Input: part model. Units: mm. Frame: model coordinates. Face numbers are marked on the shaded views. A direction names the side the tool comes from. Give positions to 0.01 mm unless a question says otherwise; leave off trailing zeros. Write each loop counter-clockwise with the first axis right and the second up, starting at its lowest first coordinate (ties: lowest second). Pieces come first, ordered by that corner, then holes. Notation, with made-up numbers: (-11.5, -4.75) -> (22.5, -4.75) arc R5 ccw to (22.5, 3.25) -> close; hole circle Ø1 at (57.25, 69.5). An arc over 180 degrees is marked (long way). Return JSON: item names as keys, results as strings. Group by question number.
Item 1: Section B-B, the plane x = 1.5. Return loops of the section in (y, z), then the cut area to 3 significant figures.
Item 2: Section D-D, the plane y = -15. Return loops of the section in (x, z), then the cut area to 3 significant figures.
Item 3: Pin query (flat end, axial travel): P1, Ø1.2, axis at y = -24, z = 3, coming from the +X side; P2, Ø0.8, axis at y = -27, z = 5.5, coming from the +X side; P3, Ø0.5, axis at x = 25, z = 5.5, coming from the -Y side; P4, Ø3, axis at x = 26, y = -1, coming from the -Z side. Return the tip coordinate at first contact, or that it passes through.
Item 4: Section C-C, the plane x = 24. Return loops of the section in (y, z), then the cut area to 3 significant figures.
Item 5: Set-up query: the marked faces 1 and 2. Return all of +Z, -Z, +X, -X, +Y, -Y with unobstructed straight access to the full face (end or side cutting, diameter ignored); none if empty.
Item 6: Section A-A, the plane z = 3.55. Return loops of the section in (x, y).
Item 7: Line query: line 1 (X direction, y = 0.5, z = 4.8); line 2 (Z direction, x = 10, y = -20); line 3 (Y direction, x = 28, z = 3.15). Output: solid intervals per line, ascending. Write a range as [from, to].
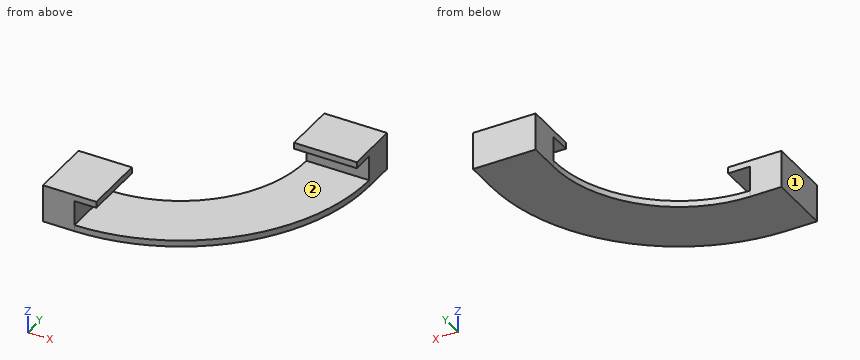
from build123d import *

# Parameters (mm, degrees)
F1_DEPTH = 1
F2_W     = 10
F2_H     = 5
F2_W_2   = 5
F2_H_2   = 10
F3_DEPTH = 5
F5_W     = 10
F5_H     = 1
F6_DEPTH = 3.5
F4_W     = 10
F4_H     = 1
F7_DEPTH = 3.5


with BuildPart() as f1:
    # F0 (on Top) → F1 (new body)
    with BuildSketch(Plane.XY):
        with BuildLine():
            Line((30, 0), (20, 0))
            ThreePointArc((20, 0), (14.1421356237, -14.1421356237), (0, -20))
            Line((0, -20), (0, -25))
            Line((0, -25), (0, -30))
            ThreePointArc((0, -30), (21.2132034356, -21.2132034356), (30, 0))
        make_face()
        with BuildLine():
            Line((20, 5), (20, 0))
            Line((20, 0), (30, 0))
            ThreePointArc((30, 0), (29.8949156836, 2.5087878084), (29.5803989155, 5))
            Line((29.5803989155, 5), (20, 5))
        make_face()
        with BuildLine():
            Line((0, -25), (0, -20))
            Line((0, -20), (-5, -20))
            Line((-5, -20), (-5, -29.5803989155))
            ThreePointArc((-5, -29.5803989155), (-2.5087878084, -29.8949156836), (0, -30))
            Line((0, -30), (0, -25))
        make_face()
        with BuildLine():
            ThreePointArc((29.5803989155, 5), (29.8949156836, 2.5087878084), (30, 0))
            Line((30, 0), (30, 5))
            Line((30, 5), (29.5803989155, 5))
        make_face()
        with BuildLine():
            Line((-5, -30), (0, -30))
            ThreePointArc((0, -30), (-2.5087878084, -29.8949156836), (-5, -29.5803989155))
            Line((-5, -29.5803989155), (-5, -30))
        make_face()
    extrude(amount=F1_DEPTH)

    # F2 (on face) → F3 (join)
    with BuildSketch(Plane.XY.offset(1)):
        with Locations((25, 2.5)):
            Rectangle(F2_W, F2_H)
        with Locations((-2.5, -25)):
            Rectangle(F2_W_2, F2_H_2)
    extrude(amount=F3_DEPTH)

    # F5 (on face) → F6 (join)
    with BuildSketch(Plane.YZ):
        with Locations((-25, 5.5)):
            Rectangle(F5_W, F5_H)
    extrude(amount=F6_DEPTH)

    # F4 (on face) → F7 (join)
    with BuildSketch(Plane.XZ):
        with Locations((25, 5.5)):
            Rectangle(F4_W, F4_H)
    extrude(amount=F7_DEPTH)


solid = f1.part
Answer below:
{
 "1": {"outline": "(-30, 5) -> (-20, 5) -> (-20, 6) -> (-30, 6) -> close; (-29.96, 0) -> (-19.94, 0) -> (-19.94, 1) -> (-29.96, 1) -> close", "area": "20.0 mm2"},
 "2": {"outline": "(13.23, 0) -> (25.98, 0) -> (25.98, 1) -> (13.23, 1) -> close", "area": "12.8 mm2"},
 "3": {"P1": "stops at x = 0", "P2": "stops at x = 3.5", "P3": "stops at y = -3.5", "P4": "stops at z = 0"},
 "4": {"outline": "(-18, 0) -> (5, 0) -> (5, 6) -> (-3.5, 6) -> (-3.5, 5) -> (0, 5) -> (0, 1) -> (-18, 1) -> close", "area": "51.5 mm2"},
 "5": {"face 1": "+Z, -Z, -X, +Y, -Y", "face 2": "+X, -Y"},
 "6": {"outline": "(-5, -30) -> (0, -30) -> (0, -20) -> (-5, -20) -> close; (20, 0) -> (30, 0) -> (30, 5) -> (20, 5) -> close"},
 "7": {"line 1": "x = [20, 30]", "line 2": "z = [0, 1]", "line 3": "y = [0, 5]"}
}
